Verification items for this drawing (mm, ordinates from the low corner). A direction names the side the tool comes from. Round coordinates to 2 decimals unless told otherwise and drop trailing zeros. Loops run counter-clockwise (first coordinate to the right, second up) from the corner with the lowest first, then second, coordinate; pieces in that order, holes last. Notation, with made-up numbers: (14, -21) -> (18, -21) arc R22 ccw to (18, 6) -> close; hole circle Ø4 at (-40, 35). An arc over 180 degrees is marked (long way). One line per item, written item: value. Start each with the question number.
1. Material ranges on L1, parallel to Y at x = 68.5, z = 66; L2, parallel to X at y = 26.5, z = 6; L3, parallel to Z at x = 45, y = 26, recorded low to high.
2. Release check for a two-part mould opening along Y. For the marked faces 6, 7, 8 and 9 record: +Y half, -Y half, draft (parallel to the pull), parting line (faces both ways), or undercut.
3. Cross-section at B-B on y = 60. Record the cut outline in (x, z), then the cut area to 3 significant figures.
4. Cross-section at C-C on z = 30.5. Record the cut outline in (x, y), then the cut area to 3 significant figures.
5. Go/stop test with flat-tipped pins: pin 1 (8 mm diameter, centred on y = 16.5, z = 42, fed in from -X); pin 2 (13 mm diameter, centred on x = 53.5, z = 82.5, fed in from +Y); pin 3 (6 mm diameter, centred on y = 40, z = 7, fed in from +X); pin 4 (4 mm diameter, centred on x = 67, y = 68.5, fed in from -Z). Record where each tip stops, or that it passes through.
6. Set-up check for the marked faces 1, 2, 3, 4 and 5: record each of +Z, -Z, +X, -X, +Y, -Y from which the full face is reachable in a straight line by a thin tool's end or side.
7. Cross-section at D-D on x = 19. Record the cut outline in (y, z).
8. Cross-section at A-A on x = 45. Record the cut outline in (y, z), then the cut area to 3 significant figures.
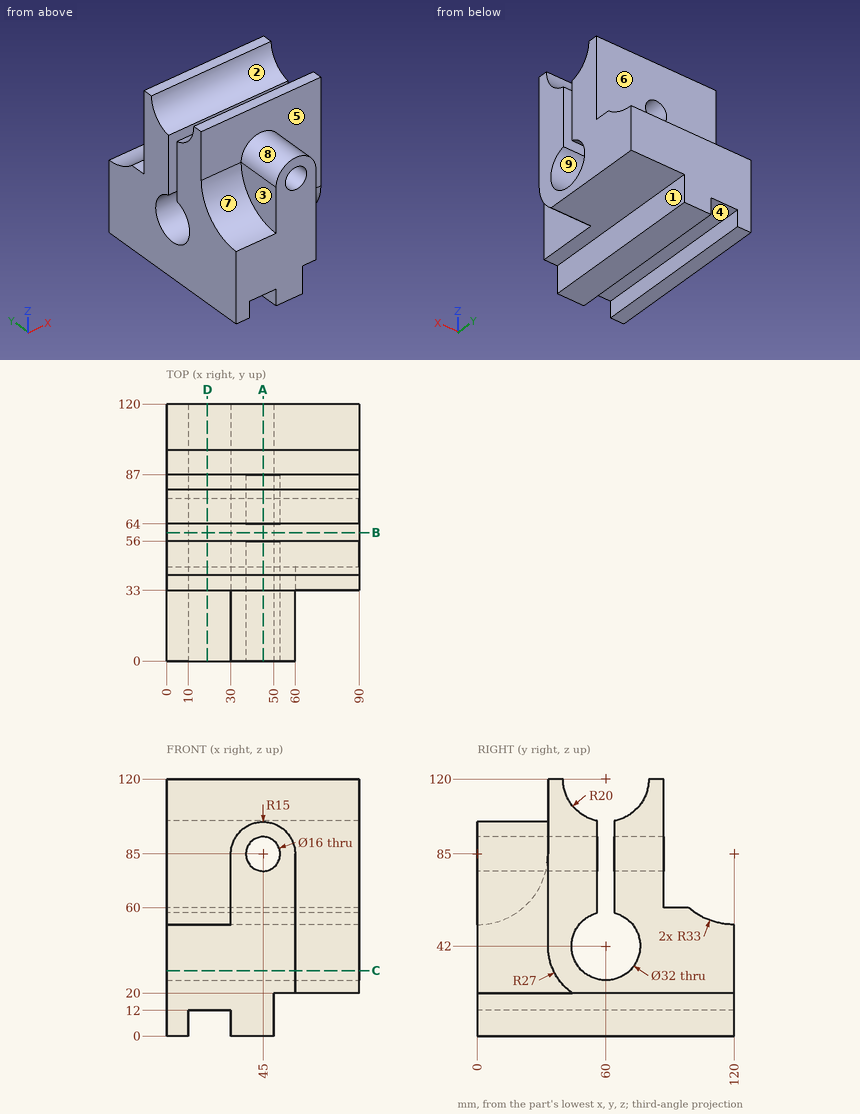
Taken from the geometry:
1. L1: y = 33 to 56, 64 to 87
1. L2: x = 0 to 10, 30 to 50
1. L3: z = 0 to 77, 93 to 100
2. face 6: +Y half
2. face 7: -Y half
2. face 8: draft
2. face 9: undercut
3. outline: (0, 0) -> (10, 0) -> (10, 12) -> (30, 12) -> (30, 0) -> (50, 0) -> (50, 20) -> (90, 20) -> (90, 26) -> (0, 26) -> close
3. area: 1,300 mm2
4. outline: (0, 0) -> (60, 0) -> (60, 35.57) -> (90, 35.57) -> (90, 48.88) -> (0, 48.88) -> close; (0, 71.12) -> (90, 71.12) -> (90, 120) -> (0, 120) -> close
4. area: 7,730 mm2
5. pin 1: stops at x = 0
5. pin 2: stops at y = 87
5. pin 3: stops at x = 50
5. pin 4: stops at z = 20
6. face 1: -Z, +X, +Y, -Y
6. face 2: +Z, +X, -X
6. face 3: +Z, -X, -Y
6. face 4: -Z, +Y, -Y
6. face 5: +Z, -Y
7. outline: (0, 12) -> (120, 12) -> (120, 52) arc R33 cw to (98.46, 60) -> (87, 60) -> (87, 120) -> (80, 120) arc R20 cw to (64, 100.4) -> (64, 57.49) arc R16 cw (long way) to (56, 57.49) -> (56, 100.4) arc R20 cw to (40, 120) -> (33, 120) -> (33, 85) arc R33 cw to (0, 52) -> close
8. outline: (0, 0) -> (120, 0) -> (120, 52) arc R33 cw to (98.46, 60) -> (87, 60) -> (87, 77) -> (64, 77) -> (64, 57.49) arc R16 cw (long way) to (56, 57.49) -> (56, 77) -> (0, 77) -> close; (0, 93) -> (56, 93) -> (56, 100.4) arc R20 cw to (40, 120) -> (33, 120) -> (33, 100) -> (0, 100) -> close; (64, 93) -> (87, 93) -> (87, 120) -> (80, 120) arc R20 cw to (64, 100.4) -> close
8. area: 8,610 mm2
